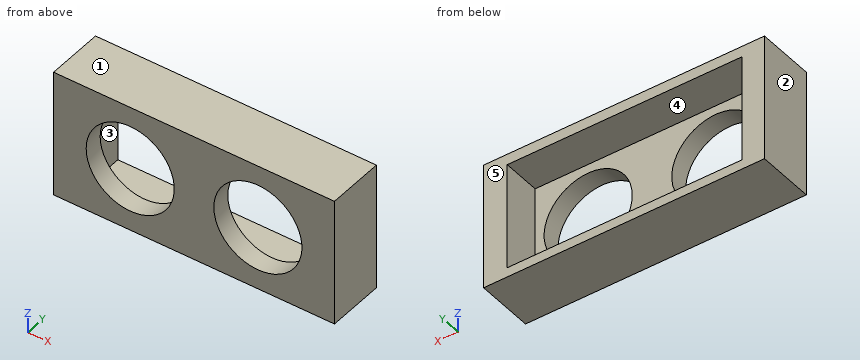
from build123d import *

# Parameters (mm, degrees)
F0_W     = 55.88
F0_H     = 25.4
F1_DEPTH = 11.43
F2_R     = 8.763
F3_DEPTH = 25.4
F4_W     = 46.736
F4_H     = 21.336
F4_R     = 8.763
F5_DEPTH = 7.62


with BuildPart() as f1:
    # F0 (on Front) → F1 (new body)
    with BuildSketch(Plane.XZ):
        with Locations((-6.981825, 4.291174)):
            Rectangle(F0_W, F0_H)
    extrude(amount=F1_DEPTH)

    # F2 (on face) → F3 (cut)
    with BuildSketch(Plane(origin=(0, 0, 0), x_dir=(-1, 0, 0), z_dir=(0, 1, 0))):
        with Locations((19.681825, 4.291174)):
            Circle(F2_R)
        with Locations((-5.718175, 4.291174)):
            Circle(F2_R)
    extrude(amount=-F3_DEPTH, mode=Mode.SUBTRACT)

    # F4 (on face) → F5 (cut)
    with BuildSketch(Plane(origin=(0, 0, 0), x_dir=(-1, 0, 0), z_dir=(0, 1, 0))):
        with Locations((7.108825, 4.164174)):
            Rectangle(F4_W, F4_H)
        with Locations((-5.718175, 4.291174)):
            Circle(F4_R, mode=Mode.SUBTRACT)
        with Locations((19.681825, 4.291174)):
            Circle(F4_R, mode=Mode.SUBTRACT)
    extrude(amount=-F5_DEPTH, mode=Mode.SUBTRACT)


solid = f1.part
Verification items for the finished model (mm, model axes). Face numbers are marked on the shaded views. A direction names the side the tool comes from. Coordinates: 2 decimals unless noted, no trailing zeros. Write each loop counter-clockwise with the first axis right and the second up, starting at its lowest first coordinate (ties: lowest second). Pieces come first, ordered by that corner, then holes. Notation, with made-up numbers: M 55.25,71 L 93.25,71 A34 ccw 93.25,103 Z; hole C 36.25,87.5 d9. An arc over 180 degrees is marked long. Use a Markdown table: item, result.
Q1. Sectioned sample at A-A, the plane y = -5.25. Record the boundary of the cut face in (x, z).
Reply:
| item | result |
|---|---|
| outline | M -34.92,-8.41 L 20.96,-8.41 L 20.96,16.99 L -34.92,16.99 Z; hole M -30.48,-6.5 L 16.26,-6.5 L 16.26,14.83 L -30.48,14.83 Z |
Q2. Set-up check for the marked faces 4 and 5: record each of +Z, -Z, +X, -X, +Y, -Y from which the full face is reachable in a straight line by a thin tool's end or side.
Reply:
| item | result |
|---|---|
| face 4 | +Y |
| face 5 | +Z, -Z, +X, -X, +Y |
Q3. Sectioned sample at B-B, the plane z = 9. Record the boundary of the cut face in (x, y), plus the area to 3 significant figures.
Reply:
| item | result |
|---|---|
| outline | M -34.92,-11.43 L -27.07,-11.43 L -27.07,-7.62 L -30.48,-7.62 L -30.48,0 L -34.92,0 Z; M -12.29,-11.43 L -1.67,-11.43 L -1.67,-7.62 L -12.29,-7.62 Z; M 13.11,-11.43 L 20.96,-11.43 L 20.96,0 L 16.26,0 L 16.26,-7.62 L 13.11,-7.62 Z |
| area | 170 mm² |
Q4. Go/stop test with flat-tipped pins: P1, Ø14, axis at x = -19.68, z = 4.29, coming from the +Y side; P2, Ø10.5, axis at x = 0, z = 1, coming from the +Y side. Record where each tip stops, or that it passes through.
Reply:
| item | result |
|---|---|
| P1 | passes through |
| P2 | stops at y = -7.62 |
Q5. Thickness scan on line 1 (X direction, y = -10, z = 4); line 2 (Z direction, x = -12, y = -2); line 3 (X direction, y = -0.5, z = -6). Record the ranges inside material, lowest first.
Reply:
| item | result |
|---|---|
| line 1 | x = -34.92 to -28.44, -10.92 to -3.04, 14.48 to 20.96 |
| line 2 | z = -8.41 to -6.5, 14.83 to 16.99 |
| line 3 | x = -34.92 to -30.48, 16.26 to 20.96 |
Q6. Sectioned sample at C-C, the plane x = -20. Record the boundary of the cut face in (y, z).
Reply:
| item | result |
|---|---|
| outline | M -11.43,-8.41 L 0,-8.41 L 0,-6.5 L -7.62,-6.5 L -7.62,-4.47 L -11.43,-4.47 Z; M -11.43,13.05 L -7.62,13.05 L -7.62,14.83 L 0,14.83 L 0,16.99 L -11.43,16.99 Z |
Q7. Draft check along Z on the marked faces 1, 2 and 3. Enter one of: +Z half, -Z half, draft (parallel to the pull), parting line (faces both ways), or undercut.
Reply:
| item | result |
|---|---|
| face 1 | +Z half |
| face 2 | draft |
| face 3 | undercut |
Q8. Sectioned sample at D-D, the plane x = -5.5. Record the boundary of the cut face in (y, z), plus the area to 3 significant figures.
Reply:
| item | result |
|---|---|
| outline | M -11.43,-8.41 L 0,-8.41 L 0,-6.5 L -7.62,-6.5 L -7.62,14.83 L 0,14.83 L 0,16.99 L -11.43,16.99 Z |
| area | 128 mm² |
